Autodesk Inventor part; units mm, degrees
ref_plane "Plano de trabajo1" through (106, -5, -152) normal (0, 0, -1) x (-1, 0, 0)
ref_plane "Plano de trabajo2" through (-50, -5, -157) normal (1, 0, 0) x (0, 0, -1)
ref_plane "YZ Plane" through (0, 0, 0) normal (1, 0, 0) x (0, 1, 0)
sketch "Boceto1" plane through (0, 0, 0) normal (0, 0, 1) x (1, 0, 0)
  line L0 (0, 0) -> (100, 0)
  line L1 (0, 300.0017) -> (0, 100.0017)
  line L2 (0, 0) -> (101, 0)
  line L3 (101, 0) -> (101, 400)
  line L4 (101, 400) -> (0, 400)
  line L5 (0, 300.0017) -> (0, 100.0017)
  line L6 (0, 0) -> (98.1777, 0) construction
  line L7 (98.1777, 0) -> (98.1777, 330) construction
  line L8 (98.1777, 330) -> (0, 330) construction
  line L9 (0, 330) -> (0, 0) construction
  line L10 (0, 300.0017) -> (-100, 300.0017) construction
  line L11 (-100, 300.0017) -> (-100, 100.0017) construction
  line L12 (-100, 100.0017) -> (0, 100.0017) construction
  line L13 (0, 100.0017) -> (0, 300.0017) construction
  line L14 (0, 300.0017) -> (-100, 300.0017)
  line L15 (-100, 300.0017) -> (-100, 100.0017)
  line L16 (-100, 100.0017) -> (0, 100.0017)
  line L17 (0, 100.0017) -> (0, 300.0017)
  line L18 (-100, 0) -> (-201, 0)
  line L19 (-201, 0) -> (-201, 400)
  line L20 (-201, 400) -> (-100, 400)
  line L21 (-100, 300.0017) -> (-100, 100.0017)
  line L22 (-100, 0) -> (0, 0)
  line L23 (-100, 400) -> (0, 400)
  line L24 (-95, 105.0017) -> (-5, 105.0017)
  line L25 (-5, 105.0017) -> (-5, 295.0017)
  line L26 (-5, 295.0017) -> (-95, 295.0017)
  line L27 (-95, 295.0017) -> (-95, 105.0017)
  line L28 (106, 400) -> (106, -5)
  line L29 (106, -5) -> (-206, -5)
  line L30 (-206, -5) -> (-206, 400)
  line L31 (-206, 400) -> (-201, 400)
  line L32 (101, 400) -> (106, 400)
  line L33 (-100, 100.0017) -> (-100, 0) construction
  line L34 (-50, -5) -> (-50, -75) construction
  line L35 (-56.35, -74.8888) -> (-43.65, -74.8888)
  line L36 (-43.65, -74.8888) -> (-38.65, -74.8888)
  line L37 (-56.35, -74.8888) -> (-61.35, -74.8888)
  arc A0 (-61.35, -74.8888) -> (-206, -5) centre (-206.1755, -189.9999) ccw
  arc A1 (106, -5) -> (-38.65, -74.8888) centre (106.1755, -189.9999) ccw
  line L38 (-38.65, -74.8888) -> (-38.65, -69.8888)
  line L39 (-61.35, -74.8888) -> (-61.35, -69.8888)
  arc A2 (-61.35, -69.8888) -> (-201, 0) centre (-206.2343, -184.9259) ccw
  arc A3 (98.1777, 0) -> (-38.65, -69.8888) centre (106.3177, -184.8208) ccw
  line L40 (-61.35, -69.8888) -> (-38.65, -69.8888)
  line L41 (-100, 0) -> (-100, -33.4687)
  line L42 (0, 0) -> (0, -33.4222)
  line L43 (-100, 400) -> (-100, 300.0017) construction
  dimension "d2" = 101
  dimension "d9" = 101
  dimension "d11" = 400
  dimension "d12" = 100
  dimension "d13" = 200
  dimension "d14" = 100
  dimension "d15" = 5
  dimension "d16" = 5
  dimension "d17" = 5
  dimension "d18" = 5
  dimension "d19" = 5
  dimension "d20" = 5
  dimension "d22" = 70
  dimension "d23" = 12.7
  dimension "d24" = 6.35
  dimension "d27" = 302
  dimension "d28" = 5
  dimension "d29" = 5
  dimension "d30" = 185
  dimension "d31" = 185
  dimension "d32" = 5
  dimension "d33" = 5
  dimension "d34" = 185
  dimension "d35" = 185
  dimension "d36" = 5
extrude "Extrusión1" add sketch "Boceto1" against normal blind 152 contours L0 A3 L29 L42 | L0 L2 L3 L32 L28 L29 A3 | L41 L29 A2 L18 | L29 A3 L42 | L29 A1 L38 A3 | A2 L29 L30 L31 L19 | L41 A2 L29 | A2 L39 A0 L29 | L38 L36 L35 L37 L39 L40 | L1 L16 L15 L14
sketch "Boceto2" plane through (0, 0, 0) normal (0, 0, 1) x (1, 0, 0)
  line L0 (-206, 400) -> (-206, -5)
  line L1 (106, -5) -> (106, 400)
  arc A0 (106, -5) -> (-38.65, -74.8888) centre (106.1755, -189.9999) ccw
  arc A1 (-61.35, -74.8888) -> (-206, -5) centre (-206.1755, -189.9999) ccw
  line L2 (-61.35, -74.8888) -> (-38.65, -74.8888)
  line L3 (-206, 400) -> (106, 400)
  line L4 (-201, 0) -> (-201, 400)
  line L5 (0, 300.0017) -> (-100, 300.0017)
  line L6 (0, 100.0017) -> (0, 300.0017)
  line L7 (-95, 105.0017) -> (-95, 295.0017)
  line L8 (-5, 295.0017) -> (-5, 105.0017)
  line L9 (-5, 105.0017) -> (-95, 105.0017)
  line L10 (-95, 295.0017) -> (-5, 295.0017)
  point P0 (0, 0)
extrude "Extrusión2" add sketch "Boceto2" along normal blind 5
ref_plane "Plano de trabajo1" through (106, -5, -152) normal (0, 0, -1) x (-1, 0, 0)
sketch "Boceto5" plane through (106, -5, -152) normal (0, 0, -1) x (-1, 0, 0)
  line L0 (312, 0) -> (312, 405)
  line L1 (312, 405) -> (307, 405)
  line L2 (5, 405) -> (307, 405)
  line L3 (5, 405) -> (0, 405)
  line L4 (0, 405) -> (0, 0)
  arc A0 (144.65, -69.8888) -> (0, 0) centre (-0.1755, -184.9999) ccw
  line L5 (144.65, -69.8888) -> (167.35, -69.8888)
  arc A1 (312, 0) -> (167.35, -69.8888) centre (312.1755, -184.9999) ccw
  line L6 (201, 110.0017) -> (111, 110.0017)
  line L7 (111, 110.0017) -> (111, 300.0017)
  line L8 (111, 300.0017) -> (201, 300.0017)
  line L9 (201, 300.0017) -> (201, 110.0017)
  point P0 (106, 5)
extrude "Extrusión3" add sketch "Boceto5" along normal blind 5
sketch "Boceto6" plane through (-61.35, -74.8888, 5) normal (0, -1, 0) x (1, 0, 0)
  line L0 (-144.65, -162) -> (167.35, -162) construction
  line L1 (11.35, -162) -> (11.35, -25.687) construction
  line L2 (0, -5) -> (0, -157) construction
  line L3 (0, -81) -> (22.7, -81) construction
  line L4 (22.7, -5) -> (22.7, -157) construction
  circle A0 centre (11.35, -81) radius 6.35
  point P0 (61.35, -5)
  dimension "d76" = 12.7
extrude "Extrusión4" cut sketch "Boceto6" against normal blind 5
sketch "Boceto7" plane through (-206, -5, 5) normal (-1, 0, 0) x (0, 0, 1)
  line L0 (-162, 0) -> (0, 0) construction
  line L1 (-81, 0) -> (-81, 5) construction
  line L2 (-81, 5) -> (-81, 35) construction
  line L3 (-81, 35) -> (-81, 115) construction
  line L4 (-81, 115) -> (-81, 145) construction
  line L5 (-81, 145) -> (-81, 225) construction
  line L6 (-81, 225) -> (-81, 255) construction
  line L7 (-81, 255) -> (-81, 335) construction
  line L8 (-157, 35) -> (-5, 35)
  line L9 (-5, 35) -> (-5, 115)
  line L10 (-5, 115) -> (-157, 115)
  line L11 (-157, 115) -> (-157, 35)
  line L12 (0, 405) -> (0, 0)
  line L13 (-162, 0) -> (-162, 405)
  line L14 (-5, 225) -> (-157, 225)
  line L15 (-157, 225) -> (-157, 145)
  line L16 (-157, 145) -> (-5, 145)
  line L17 (-5, 145) -> (-5, 225)
  line L18 (-5, 335) -> (-157, 335)
  line L19 (-157, 335) -> (-157, 255)
  line L20 (-157, 255) -> (-5, 255)
  line L21 (-5, 255) -> (-5, 335)
  point P0 (-5, 5)
  dimension "d47" = 5
  dimension "d48" = 30
  dimension "d49" = 80
  dimension "d50" = 30
  dimension "d51" = 80
  dimension "d52" = 30
  dimension "d53" = 80
  dimension "d54" = 5
  dimension "d55" = 5
  dimension "d58" = 110
sketch "Boceto8" plane through (106, -5, 5) normal (1, 0, 0) x (0, 0, -1)
  line L0 (5, 335) -> (157, 335)
  line L1 (157, 335) -> (157, 255)
  line L2 (157, 255) -> (5, 255)
  line L3 (5, 255) -> (5, 335)
  line L4 (5, 225) -> (157, 225)
  line L5 (157, 225) -> (157, 145)
  line L6 (157, 145) -> (5, 145)
  line L7 (5, 145) -> (5, 225)
  line L8 (5, 115) -> (157, 115)
  line L9 (157, 115) -> (157, 35)
  line L10 (157, 35) -> (5, 35)
  line L11 (5, 35) -> (5, 115)
  point P0 (5, 5)
extrude "Extrusión5" cut sketch "Boceto7" against normal blind 5
extrude "Extrusión6" cut sketch "Boceto8" against normal blind 5
sketch "Boceto9" plane through (106, -5, -152) normal (0, 0, 1) x (1, 0, 0)
  line L0 (0, 405) -> (0, 0) construction
  line L1 (0, 372.4568) -> (-312, 372.4568) construction
  line L2 (-312, 0) -> (-312, 405) construction
  line L3 (-156, 372.4568) -> (-156, 300.0017) construction
  line L4 (-111, 300.0017) -> (-201, 300.0017) construction
  line L5 (-312, 405) -> (0, 405) construction
  line L6 (-156, 405) -> (-156, 385) construction
  line L7 (-106, 405) -> (-106, 305) construction
  line L8 (-106, 305) -> (-206, 305) construction
  line L9 (-206, 305) -> (-106, 305)
  line L10 (-206, 305) -> (-156, 367.45)
  line L11 (-106, 305) -> (-156, 367.45)
  point P0 (-106, 5)
  dimension "d71" = 20
  dimension "d72" = 100
  dimension "d73" = 80
extrude "Extrusión7" add sketch "Boceto9" along normal blind 152
thread "Rosca1"
sketch "Boceto11" plane through (106, -5, 5) normal (1, 0, 0) x (0, 0, -1)
  line L0 (157, 405) -> (157, 335)
  line L1 (5, 350) -> (157, 350)
  line L2 (157, 350) -> (157, 365)
  line L3 (157, 365) -> (5, 365)
  line L4 (5, 365) -> (5, 350)
  line L5 (5, 105.0017) -> (5, 305.0017)
  line L6 (5, 10) -> (157, 10)
  line L7 (157, 10) -> (157, 25)
  line L8 (157, 25) -> (5, 25)
  line L9 (5, 25) -> (5, 10)
  line L10 (162, 405) -> (0, 405)
  line L11 (157, 35) -> (5, 35)
  line L12 (0, 405) -> (0, 0)
  line L13 (5, 122.5) -> (0, 122.5)
  line L14 (0, 122.5) -> (0, 137.5)
  line L15 (0, 137.5) -> (5, 137.5)
  line L16 (5, 137.5) -> (5, 122.5)
  line L17 (5, 232.5) -> (0, 232.5)
  line L18 (0, 232.5) -> (0, 247.5)
  line L19 (0, 247.5) -> (5, 247.5)
  line L20 (5, 247.5) -> (5, 232.5)
  line L21 (157, 255) -> (5, 255)
  line L22 (5, 225) -> (157, 225)
  line L23 (157, 145) -> (5, 145)
  line L24 (5, 115) -> (157, 115)
  point P0 (5, 5)
  dimension "d79" = 152
  dimension "d80" = 40
  dimension "d81" = 15
  dimension "d84" = 15
  dimension "d89" = 10
  dimension "d92" = 7.5
  dimension "d93" = 7.5
  dimension "d94" = 7.5
  dimension "d95" = 7.5
extrude "Extrusión8" add sketch "Boceto11" along normal blind 3 contours L0 L1 L4 L3 | L19 L5 L17 L12 | L15 L5 L13 L12 | L9 L8 L7 L6
sketch "Boceto12" plane through (106, 345, -152) normal (0, -1, 0) x (1, 0, 0)
  line L0 (1, 152) -> (2, 152)
  line L1 (2, 152) -> (2, 0)
  line L2 (2, 0) -> (1, 0)
  line L3 (1, 0) -> (1, 152)
  line L4 (0, 152) -> (0, 0)
  line L5 (0, 152) -> (3, 152)
  line L6 (0, 0) -> (3, 0)
  point P0 (-106, 152)
  dimension "d96" = 1
  dimension "d97" = 1
  dimension "d98" = 0
  dimension "d99" = 0
extrude "Extrusión9" cut sketch "Boceto12" against normal blind 5 contours L0 L1 L2 L3
sketch "Boceto13" plane through (106, 20, 0) normal (0, 1, 0) x (1, 0, 0)
  line L0 (2, 0) -> (1, 0)
  line L1 (1, 0) -> (1, 152)
  line L2 (1, 152) -> (2, 152)
  line L3 (2, 152) -> (2, 0)
  line L4 (0, 0) -> (3, 0)
  line L5 (0, 0) -> (0, 152)
  line L6 (0, 152) -> (3, 152)
  point P0 (-106, 0)
  dimension "d102" = 0
  dimension "d103" = 1
  dimension "d104" = 1
  dimension "d105" = 0
extrude "Extrusión10" cut sketch "Boceto13" against normal blind 5 contours L0 L1 L2 L3
ref_plane "Plano de trabajo2" through (-50, -5, -157) normal (1, 0, 0) x (0, 0, -1)
mirror "Simetría1" about plane through (-50, -5, -157) normal (1, 0, 0) of "Extrusión8"
sketch "Boceto14" plane through (-206, 20, 0) normal (0, 1, 0) x (1, 0, 0)
  line L0 (-2, 152) -> (-1, 152)
  line L1 (-1, 152) -> (-1, 0)
  line L2 (-1, 0) -> (-2, 0)
  line L3 (-2, 0) -> (-2, 152)
  line L4 (0, 152) -> (-3, 152)
  line L5 (-3, 152) -> (-3, 0)
  line L6 (0, 0) -> (-3, 0)
  point P0 (206, 0)
  dimension "d108" = 0
  dimension "d109" = 1
  dimension "d110" = 1
  dimension "d111" = 0
extrude "Extrusión11" cut sketch "Boceto14" against normal blind 5 contours L0 L1 L2 L3
sketch "Boceto15" plane through (-206, 345, -152) normal (0, -1, 0) x (1, 0, 0)
  line L0 (-1, 0) -> (-2, 0)
  line L1 (-2, 0) -> (-2, 152)
  line L2 (-2, 152) -> (-1, 152)
  line L3 (-1, 152) -> (-1, 0)
  line L4 (0, 0) -> (-3, 0)
  line L5 (-3, 0) -> (-3, 152)
  line L6 (0, 152) -> (-3, 152)
  point P0 (206, 152)
  dimension "d114" = 0
  dimension "d115" = 1
  dimension "d116" = 1
  dimension "d117" = 0
extrude "Extrusión12" cut sketch "Boceto15" against normal blind 5 contours L0 L1 L2 L3
equation "\"d16\" = d15"
equation "\"d17\" = d15"
equation "\"d18\" = d15"
equation "\"d19\" = d15"
equation "\"d20\" = d15"
equation "\"d24\" = 0.5 * d23"
equation "\"d31\" = d30"
equation "\"d84\" = d81"
properties part number "Contenedor" material "Acrílico, claro"
Work out the finished part from the listing and answer in its coordinate system (mm). A direction names the side the tool comes from. Give positions to 0.01 mm unless a question says otherwise; leave off trailing zeros. Order: outer loops, then holes, each group sorted by start corner. A loop starts at its lowest first (then second) coordinate and runs counter-clockwise, first axis right, second up. Notation, with made-up numbers: M 66.5,59.5 L 120.5,59.5 A22 ccw 120.5,84.5 Z; hole C 31.5,53 d7. An arc over 180 degrees is marked long. Return JSON: item names as keys, results as strings.
Q1. The mould has two halves that part along Z. Classify faces 4 (the face through (26.74, -22.92, -154.46)), 5 (the face through (-51.38, -72.42, -82.2)): pulls with the +Z half, pulls with the -Z half, needs draft (parallel to the pull), parting line crosses it, or undercut.
Answer below:
{"face 4": "needs draft", "face 5": "undercut"}
Q2. Each of these flat-tipped pins is pushed along its axis until it touches: pin 1 (12 mm diameter, centred on x = 18, z = -74, fed in from -Y); pin 2 (12 mm diameter, centred on x = -37.5, z = -43, fed in from +Y); pin 3 (4 mm diameter, centred on y = 250.5, z = -139.5, fed in from +X). Where does it stop, or does it pass through?
Answer below:
{"pin 1": "stops at y = -30.76", "pin 2": "stops at y = 354.33", "pin 3": "stops at x = 106"}
Q3. Find section A-A, the plane y = 201. Write down the section's boundary in (x, z), and give its area (3 significant figures).
Answer below:
{"outline": "M -206,-157 L -95,-157 L -95,5 L -206,5 L -206,0 L -100,0 L -100,-152 L -206,-152 Z; M -5,-157 L 106,-157 L 106,-152 L 0,-152 L 0,0 L 106,0 L 106,5 L -5,5 Z", "area": "3,740 mm^2"}
Q4. Find section B-B, the plane z = -140. State how many separate pieces and enclosed holes the cut face has, and give its area (3 significant figures).
Answer below:
{"separate pieces": "8", "enclosed holes": "1", "area": "11,600 mm^2"}
Q5. Which of the six approach directions +Z, -Z, +X, -X, +Y, -Y give full straight-line access (tool end or side, diameter ignored) to faces 1 (the face through (-100, -17, -75)), 2 (the face through (-75.35, 330.79, -77.06)), 3 (the face through (109, 353, -75))?
Answer below:
{"face 1": "none", "face 2": "+Y", "face 3": "+Z, -Z, +X, +Y, -Y"}
Q6. Find section C-C, the plane x = -163.5. Write down the section's boundary in (y, z).
Answer below:
{"outline": "M -9.99,-157 L 400,-157 L 400,-152 L 0,-152 L 0,0 L 400,0 L 400,5 L -9.99,5 Z"}
Q7. Find the intervals of material crossed by line 1 along Z through (x, y) = (-50, -71.55); line 2 along X through (y, z) = (106.5, -26); line 3 along X through (y, z) = (345.5, -124), in increasing order. Write a range as [from, to].
Answer below:
{"line 1": "z = [-157, -82.35], [-69.65, 5]", "line 2": "x = [-100, -95], [-5, 0]", "line 3": "x = [-209, -208], [-207, -201], [-63.57, -36.43], [101, 107], [108, 109]"}
